```python
from build123d import *

# Parameters (mm, degrees)
SKETCH_1_W          = 60
SKETCH_1_H          = 60
SKETCH_1_R          = 4
EXTRUDE_1_DEPTH     = 5
SKETCH_2_W          = 21.03
SKETCH_2_H          = 23.5
CUT_EXTRUDE_1_DEPTH = 86


with BuildPart() as part:
    # 草图1 → 凸台-拉伸1 (new body)
    with BuildSketch(Plane(origin=(0, 0, 0), x_dir=(1, 0, 0), z_dir=(0, 1, 0))):
        with Locations((30, -30)):
            Rectangle(SKETCH_1_W, SKETCH_1_H)
        with Locations(Location((12, -12, 0), (0, 0, 270))):
            Circle(SKETCH_1_R, mode=Mode.SUBTRACT)
    extrude(amount=EXTRUDE_1_DEPTH)

    # 草图2 → 切除-拉伸1 (cut, through all)
    with BuildSketch(Plane(origin=(0, 0, 0), x_dir=(1, 0, 0), z_dir=(0, 1, 0))):
        with Locations((10.515, -48.25)):
            Rectangle(SKETCH_2_W, SKETCH_2_H)
    extrude(amount=CUT_EXTRUDE_1_DEPTH, mode=Mode.SUBTRACT)


solid = part.part
```
Model file for the job. Use its own axes, mm. A direction names the side the tool comes from. Give positions to 0.01 mm unless a question says otherwise; leave off trailing zeros. Loops run counter-clockwise (first coordinate to the right, second up) from the corner with the lowest first, then second, coordinate; pieces in that order, holes last. Notation, with made-up numbers: (-4, 24.25) -> (18, 24.25) arc R9 ccw to (18, 37.25) -> close; hole circle Ø5 at (10.25, 67.5). An arc over 180 degrees is marked (long way). Write each question's results on one line, items separated by ' | '.
(1) Cut at B-B on y = 2.85. List the corners of the cut face in (x, z), and give its area (3 significant figures).
Geometry results:
outline: (0, 0) -> (60, 0) -> (60, 60) -> (21.03, 60) -> (21.03, 36.5) -> (0, 36.5) -> close; hole circle Ø8 at (12, 12) | area: 3,060 mm²
(2) Probe line 1 along X through (y, z) = (1.1, 12); line 2 along X through (y, z) = (1.05, 47.5); line 3 along Z through (x, y) = (6, 0.45). List the from-to ranges inside material, lowest first.
Geometry results:
line 1: x = 0 to 8, 16 to 60 | line 2: x = 21.03 to 60 | line 3: z = 0 to 36.5
(3) Pull direction Z, two halves, no side cores. Call faces 3 (the flat face through (40, 2, 60)), 4 (the cylindrical face through (14.7, 2.46, 9.05)), 5 (the flat face through (30, 2, 0)): released by +Z, released by -Z, zero draft, split by the parting line, or undercut.
Geometry results:
face 3: released by +Z | face 4: undercut | face 5: released by -Z
(4) Cut at D-D on z = 45.5. List the corners of the cut face in (x, y), and give its area (3 significant figures).
Geometry results:
outline: (21.03, 0) -> (60, 0) -> (60, 5) -> (21.03, 5) -> close | area: 195 mm²
(5) Cut at C-C on z = 12. List the corners of the cut face in (x, y), and give its area (3 significant figures).
Geometry results:
outline: (0, 0) -> (8, 0) -> (8, 5) -> (0, 5) -> close; (16, 0) -> (60, 0) -> (60, 5) -> (16, 5) -> close | area: 260 mm²
(6) Tool access for faces 1 (the flat face through (60, 2, 30)), 2 (the flat face through (21.03, 2, 48)): list every direction of +Z, -Z, +X, -X, +Y, -Y with a clear straight run to the whole face (end or side of a thin tool).
Geometry results:
face 1: +Z, -Z, +X, +Y, -Y | face 2: +Z, -X, +Y, -Y
(7) Cut at A-A on x = 12. List the corners of the cut face in (y, z).
Geometry results:
outline: (0, 0) -> (5, 0) -> (5, 8) -> (0, 8) -> close; (0, 16) -> (5, 16) -> (5, 36.5) -> (0, 36.5) -> close
